from build123d import *

# Parameters (mm, degrees)
SKETCH1_W           = 25.4
SKETCH1_H           = 152.4
BOSS_EXTRUDE1_DEPTH = 6.604
CUT_EXTRUDE1_DEPTH  = 7.604
FILLET1_R           = 6.35


with BuildPart() as part:
    # Sketch1 → Boss-Extrude1 (new body)
    with BuildSketch(Plane(origin=(0, 0, 0), x_dir=(1, 0, 0), z_dir=(0, 1, 0))):
        Rectangle(SKETCH1_W, SKETCH1_H)
    extrude(amount=BOSS_EXTRUDE1_DEPTH)

    # Sketch2 → Cut-Extrude1 (cut, through all)
    with BuildSketch(Plane(origin=(0, 6.604, 0), x_dir=(1, 0, 0), z_dir=(0, 1, 0))):
        with BuildLine():
            Line((-6.35, 59.309), (6.35, 59.309))
            ThreePointArc((6.35, 59.309), (8.509, 57.15), (6.35, 54.991))
            Line((6.35, 54.991), (-6.35, 54.991))
            ThreePointArc((-6.35, 54.991), (-8.509, 57.15), (-6.35, 59.309))
        make_face()
        with BuildLine():
            Line((-6.35, -54.991), (6.35, -54.991))
            ThreePointArc((6.35, -54.991), (8.509, -57.15), (6.35, -59.309))
            Line((6.35, -59.309), (-6.35, -59.309))
            ThreePointArc((-6.35, -59.309), (-8.509, -57.15), (-6.35, -54.991))
        make_face()
    extrude(amount=-CUT_EXTRUDE1_DEPTH, mode=Mode.SUBTRACT)

    # Fillet1
    fillet1_edges = [part.edges().sort_by_distance(p)[0] for p in [
        (-12.7, 3.302, -76.2),
        (12.7, 3.302, -76.2),
        (12.7, 3.302, 76.2),
        (-12.7, 3.302, 76.2),
    ]]
    fillet(fillet1_edges, radius=FILLET1_R)


solid = part.part
Here's how the part is built. I have some questions about the finished solid (model axes, mm). A direction names the side the tool comes from. Round coordinates to 2 decimals unless told otherwise and drop trailing zeros. Order: outer loops, then holes, each group sorted by start corner. A loop starts at its lowest first (then second) coordinate and runs counter-clockwise, first axis right, second up. Notation, with made-up numbers: (-31.5, 70.25) -> (-22.5, 70.25) arc R11 cw to (-22.5, 84.25) -> close; hole circle Ø7 at (-8, 37). An arc over 180 degrees is marked (long way). Return JSON: item names as keys, results as strings.
Q1. For pin 1 Ø1 at (x, y) = (9, 3) entering from -Z, with a flat end and sliding along its axis, tell me the tip position at first contact or that it passes through.
Filled sheet:
{"pin 1": "stops at z = -75.82"}
Q2. Which directions (+Z, -Z, +X, -X, +Y, -Y) give clear straight access to the entire face, cutting with the end or side of a thin tool? Please do faces 1 (the cylindrical face through (10.79, 3.35, -74.39)), 2 (the flat face through (0, 3, -59.309)).
Filled sheet:
{"face 1": "-Z, +X, +Y, -Y", "face 2": "+Y, -Y"}
Q3. If we section it at B-B on y = 3.25: List the corners of the cut face in (x, z) for me, plus the area to 3 significant figures.
Filled sheet:
{"outline": "(-12.7, -69.85) arc R6.35 ccw to (-6.35, -76.2) -> (6.35, -76.2) arc R6.35 ccw to (12.7, -69.85) -> (12.7, 69.85) arc R6.35 ccw to (6.35, 76.2) -> (-6.35, 76.2) arc R6.35 ccw to (-12.7, 69.85) -> close; hole (-6.35, -59.31) -> (6.35, -59.31) arc R2.16 ccw to (6.35, -54.99) -> (-6.35, -54.99) arc R2.16 ccw to start; hole (-6.35, 54.99) -> (6.35, 54.99) arc R2.16 ccw to (6.35, 59.31) -> (-6.35, 59.31) arc R2.16 ccw to start", "area": "3,700 mm^2"}
Q4. If we mould it in two halves opening along X, with no side actions, what happens to faces 3 (the flat face through (0, 0, -1)), 4 (the cylindrical face through (-8.51, 3.35, 57.2)), 5 (the cylindrical face through (8.51, 3.35, -57.2)), 6 (the flat face through (-12.7, 3, 1))? For each: released by +X, released by -X, zero draft, split by the parting line, or undercut.
Filled sheet:
{"face 3": "zero draft", "face 4": "undercut", "face 5": "undercut", "face 6": "released by -X"}
Q5. If we section it at D-D on x = 11: List the corners of the cut face in (y, z) for me, plus the area to 3 significant figures.
Filled sheet:
{"outline": "(0, -74.17) -> (6.6, -74.17) -> (6.6, 74.17) -> (0, 74.17) -> close", "area": "980 mm^2"}
Q6. I need wall thicknesses on line 1 along Z through (x, y) = (3.25, 5); line 2 along Z through (x, y) = (-8.25, 2); line 3 along Z through (x, y) = (11.75, 4.25). Which ranges of each line are inside material? Lowest first, please. Write a range as from..to.
Filled sheet:
{"line 1": "z = -76.2..-59.31, -54.99..54.99, 59.31..76.2", "line 2": "z = -75.91..-58.18, -56.12..56.12, 58.18..75.91", "line 3": "z = -73.19..73.19"}
Q7. If we section it at C-C on z = -57.15: List the corners of the cut face in (x, y) for me.
Filled sheet:
{"outline": "(-12.7, 0) -> (-8.51, 0) -> (-8.51, 6.6) -> (-12.7, 6.6) -> close; (8.51, 0) -> (12.7, 0) -> (12.7, 6.6) -> (8.51, 6.6) -> close"}
Q8. If we section it at A-A on x = -4.75: List the corners of the cut face in (y, z) for me, plus the area to 3 significant figures.
Filled sheet:
{"outline": "(0, -76.2) -> (6.6, -76.2) -> (6.6, -59.31) -> (0, -59.31) -> close; (0, -54.99) -> (6.6, -54.99) -> (6.6, 54.99) -> (0, 54.99) -> close; (0, 59.31) -> (6.6, 59.31) -> (6.6, 76.2) -> (0, 76.2) -> close", "area": "949 mm^2"}
